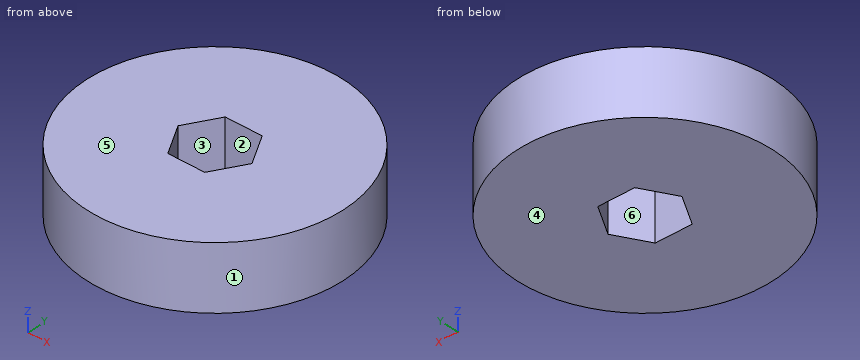
```python
from build123d import *

# Parameters (mm, degrees)
SKETCH1_R               = 25.4
BOSS_EXTRUDE1_DEPTH     = 12.7
CUT_EXTRUDE1_DEPTH      = 39.1
CUT_EXTRUDE1_DEPTH_BACK = 39.1


with BuildPart() as part:
    # Sketch1 → Boss-Extrude1 (new body)
    with BuildSketch(Plane.XY):
        Circle(SKETCH1_R)
    extrude(amount=BOSS_EXTRUDE1_DEPTH)

    # Sketch2 → Cut-Extrude1 (cut, two sides: drawn at the far end of the back side and taken through both)
    with BuildSketch(Plane.XY.offset(12.7).offset(-CUT_EXTRUDE1_DEPTH_BACK)):
        Polygon((7.332348419, 0), (3.666174209, 6.35), (-3.666174209, 6.35), (-7.332348419, 0), (-3.666174209, -6.35), (3.666174209, -6.35), align=None)
    extrude(amount=CUT_EXTRUDE1_DEPTH + CUT_EXTRUDE1_DEPTH_BACK, mode=Mode.SUBTRACT)


solid = part.part
```
Check sheet for the modelled part. Datum: model origin and axes. Units: mm. Face numbers are marked on the shaded views. A direction names the side the tool comes from. Give positions to 0.01 mm unless a question says otherwise; leave off trailing zeros. Write each loop counter-clockwise with the first axis right and the second up, starting at its lowest first coordinate (ties: lowest second). Pieces come first, ordered by that corner, then holes.
Item 1: Cross-section at D-D (x = -12.5). Enter the section's corners in (y, z).
Item 2: Cross-section at A-A (x = 0). Enter the section's corners in (y, z).
Item 3: Cross-section at B-B (z = 5.25). Enter the section's corners in (x, y), and give its area (3 significant figures).
Item 4: Access from +Z, -Z, +X, -X, +Y, -Y to the whole of each face (thin tool, end or side, straight path). Record for the marked faces 5 and 6.
Item 5: Scan lines: L1, parallel to X at y = 1, z = 7 (3 decimals); L2, parallel to Y at x = -6, z = 5.75; L3, parallel to X at y = -16, z = 7.5. Record each from-to range of solid material in increasing order.
Item 6: Gauge pin test, flat ends, axial feed: pin 1 (3.5 mm diameter, centred on x = 0.5, z = 7.5, fed in from +Y); pin 2 (1 mm diameter, centred on x = -12.5, z = 8, fed in from +Y); pin 3 (6 mm diameter, centred on y = 4.5, z = 8, fed in from +X). Record the tip position at first contact, or that the pin passes through.
Item 7: Cross-section at C-C (y = -4.5). Enter the section's corners in (x, z), and give its area (3 significant figures).
Item 8: Draft check along Y on the marked faces 1, 2, 3 and 4. Enter one of: released by +Y, released by -Y, zero draft, split by the parting line, or undercut.
Report:
1. outline: (-22.11, 0) - (22.11, 0) - (22.11, 12.7) - (-22.11, 12.7) - close
2. outline: (-25.4, 0) - (-6.35, 0) - (-6.35, 12.7) - (-25.4, 12.7) - close; (6.35, 0) - (25.4, 0) - (25.4, 12.7) - (6.35, 12.7) - close
3. outline: circle Ø50.8 at (0, 0); hole (-7.33, 0) - (-3.67, -6.35) - (3.67, -6.35) - (7.33, 0) - (3.67, 6.35) - (-3.67, 6.35) - close
3. area: 1,890 mm2
4. face 5: +Z, +X, -X, +Y, -Y
4. face 6: +Z, -Z
5. L1: x = -25.38 to -6.755, 6.755 to 25.38
5. L2: y = -24.68 to -2.31, 2.31 to 24.68
5. L3: x = -19.73 to 19.73
6. pin 1: stops at y = 25.4
6. pin 2: stops at y = 22.39
6. pin 3: stops at x = 25.36
7. outline: (-25, 0) - (-4.73, 0) - (-4.73, 12.7) - (-25, 12.7) - close; (4.73, 0) - (25, 0) - (25, 12.7) - (4.73, 12.7) - close
7. area: 515 mm2
8. face 1: split by the parting line
8. face 2: undercut
8. face 3: undercut
8. face 4: zero draft
